Input: part model. Units: mm. Frame: model coordinates. A direction names the side the tool comes from. Coordinates: 2 decimals unless noted, no trailing zeros. Loops run counter-clockwise (first coordinate to the right, second up) from the corner with the lowest first, then second, coordinate; pieces in that order, holes last. Notation, with made-up numbers: (37.25, 82) - (77.25, 82) arc R29 cw to (77.25, 117) - close; hole circle Ø5 at (-34, 16.5). An arc over 180 degrees is marked (long way). Answer as CSV lines item,"result". Start each with the question number.
```python
from build123d import *

# Parameters (mm, degrees)
SKETCH1_W           = 40.2
SKETCH1_H           = 20.2
SKETCH1_W_2         = 38.2
SKETCH1_H_2         = 18.2
BOSS_EXTRUDE1_DEPTH = 10.65
FILLET1_R           = 1
SKETCH2_W           = 39.2
SKETCH2_H           = 19.2
SKETCH2_W_2         = 38.2
SKETCH2_H_2         = 18.2
BOSS_EXTRUDE2_DEPTH = 0.5
SKETCH3_W           = 38.2
SKETCH3_H           = 18.2
BOSS_EXTRUDE3_DEPTH = 1
BOSS_EXTRUDE4_START = -21.8
SKETCH4_R           = 1.4
BOSS_EXTRUDE4_DEPTH = 21.8
SKETCH5_R           = 1
CUT_EXTRUDE1_DEPTH  = 34.690677644
SKETCH6_W           = 40.2
SKETCH6_H           = 20.2
SKETCH6_W_2         = 39.2
SKETCH6_H_2         = 19.2
CUT_EXTRUDE2_DEPTH  = 2
SKETCH7_W           = 5
SKETCH7_H           = 2
CUT_EXTRUDE3_DEPTH  = 0.5


with BuildPart() as part:
    # Sketch1 → Boss-Extrude1 (new, symmetric)
    with BuildSketch(Plane(origin=(0, 0, 0), x_dir=(1, 0, 0), z_dir=(0, 1, 0))):
        with Locations((3.133727572, 0.855166052)):
            Rectangle(SKETCH1_W, SKETCH1_H)
        with Locations((3.133727572, 0.855166052)):
            Rectangle(SKETCH1_W_2, SKETCH1_H_2, mode=Mode.SUBTRACT)
    extrude(amount=BOSS_EXTRUDE1_DEPTH, both=True)

    # Fillet1
    fillet1_edges = [part.edges().sort_by_distance(p)[0] for p in [
        (-16.966272428, 0, -10.955166052),
        (23.233727572, 0, -10.955166052),
        (23.233727572, 0, 9.244833948),
        (-16.966272428, 0, 9.244833948),
    ]]
    fillet(fillet1_edges, radius=FILLET1_R)

    # Sketch2 → Boss-Extrude2 (add)
    with BuildSketch(Plane(origin=(0, 10.65, 0), x_dir=(1, 0, 0), z_dir=(0, 1, 0))):
        with Locations((3.133727572, 0.855166052)):
            Rectangle(SKETCH2_W, SKETCH2_H)
        with Locations((3.133727572, 0.855166052)):
            Rectangle(SKETCH2_W_2, SKETCH2_H_2, mode=Mode.SUBTRACT)
    extrude(amount=BOSS_EXTRUDE2_DEPTH)

    # Sketch3 → Boss-Extrude3 (add)
    with BuildSketch(Plane(origin=(0, 10.65, 0), x_dir=(1, 0, 0), z_dir=(0, 1, 0))):
        with Locations((3.133727572, 0.855166052)):
            Rectangle(SKETCH3_W, SKETCH3_H)
    extrude(amount=-BOSS_EXTRUDE3_DEPTH)

    # Sketch4 → Boss-Extrude4 (add)
    with BuildSketch(Plane(origin=(0, 11.15, 0), x_dir=(1, 0, 0), z_dir=(0, 1, 0)).offset(BOSS_EXTRUDE4_START)):
        with Locations((-15.066272428, 9.055166052)):
            Circle(SKETCH4_R)
        with Locations((-15.066272428, -7.344833948)):
            Circle(SKETCH4_R)
        with Locations((21.333727572, 9.055166052)):
            Circle(SKETCH4_R)
        with Locations((21.133727572, -7.344833948)):
            Circle(SKETCH4_R)
    extrude(amount=BOSS_EXTRUDE4_DEPTH)

    # Sketch5 → Cut-Extrude1 (cut, through all)
    with BuildSketch(Plane(origin=(0, 11.15, 0), x_dir=(1, 0, 0), z_dir=(0, 1, 0))):
        with Locations(Location((-15.066272428, 9.055166052, 0), (0, 0, 270))):
            Circle(SKETCH5_R)
        with Locations(Location((-15.066272428, -7.344833948, 0), (0, 0, 270))):
            Circle(SKETCH5_R)
        with Locations(Location((21.333727572, 9.055166052, 0), (0, 0, 270))):
            Circle(SKETCH5_R)
        with Locations(Location((21.133727572, -7.344833948, 0), (0, 0, 270))):
            Circle(SKETCH5_R)
    extrude(amount=-CUT_EXTRUDE1_DEPTH, mode=Mode.SUBTRACT)

    # Sketch6 → Cut-Extrude2 (cut)
    with BuildSketch(Plane.XZ.offset(10.65)):
        with Locations((3.133727572, -0.855166052)):
            Rectangle(SKETCH6_W, SKETCH6_H)
        with Locations((3.133727572, -0.855166052)):
            Rectangle(SKETCH6_W_2, SKETCH6_H_2, mode=Mode.SUBTRACT)
    extrude(amount=-CUT_EXTRUDE2_DEPTH, mode=Mode.SUBTRACT)

    # Sketch7 → Cut-Extrude3 (cut)
    with BuildSketch(Plane(origin=(22.733727572, 0, 0), x_dir=(0, 0, -1), z_dir=(1, 0, 0))):
        with Locations((0.755166052, -9.65)):
            Rectangle(SKETCH7_W, SKETCH7_H)
    extrude(amount=-CUT_EXTRUDE3_DEPTH, mode=Mode.SUBTRACT)


solid = part.part
```
Item 1: Draft query along X for faces 6 (the cylindrical face through (-14.1, 10.9, -8.04)), 7 (the flat face through (3.04, 11.15, -10.14)), 8 (the flat face through (3, -1, -9.955)), 9 (the cylindrical face through (-16.681, 0.865, -10.654)). Return one class per face: pulls with the +X half, pulls with the -X half, needs draft (parallel to the pull), parting line crosses it, or undercut.
Item 2: Section query C-C, the plane x = 16. Output: boundary loops of the cut face in (y, z), and give its area (3 significant figures).
Item 3: Section query B-B, the plane y = -9.5. Give the number of separate pieces and of enclosed holes in the cut face, and give its area (3 significant figures).
Item 4: Section query A-A, the plane z = -5.25. Output: boundary loops of the cut face in (x, y).
Item 5: Section query D-D, the plane z = -9.5. Output: boundary loops of the cut face in (x, y).
Item 6: Contact query for flat-ended pins moving along their axis: P1, Ø1.6, axis at y = -9.5, z = -8.5, coming from the +X side; P2, Ø2, axis at x = 10, z = 4, coming from the +Y side; P3, Ø0.6, axis at y = -10, z = 0, coming from the -X side; P4, Ø1.2, axis at x = 21.33, z = -9.06, coming from the -Y side. Output: stop coordinate, or through.
Item 7: Set-up query: faces 1 (the flat face through (3, -10, -10.455)), 2 (the flat face through (-16.966, 1, -1)), 3 (the flat face through (3, 1, -10.955)), 4 (the flat face through (-16.466, -10, -1)), 5 (the flat face through (22.234, -1, -1)). Return all of +Z, -Z, +X, -X, +Y, -Y with unobstructed straight access to the full face (end or side cutting, diameter ignored); none if empty.
Item 8: Material intervals for probe 1 along Z at (x, y) = (15.5, 5.75); probe 2 along X at (y, z) = (-6.75, -4); probe 3 along Z at (x, y) = (14.5, -9.5), sorted ascending.
Response values:
1,face 6,"undercut"
1,face 7,"needs draft"
1,face 8,"undercut"
1,face 9,"pulls with the -X half"
2,outline,"(-10.65, -10.46) - (-8.65, -10.46) - (-8.65, -10.96) - (10.65, -10.96) - (10.65, -10.46) - (11.15, -10.46) - (11.15, -9.96) - (10.65, -9.96) - (10.65, 8.24) - (11.15, 8.24) - (11.15, 8.74) - (10.65, 8.74) - (10.65, 9.24) - (-8.65, 9.24) - (-8.65, 8.74) - (-10.65, 8.74) - (-10.65, 8.24) - (9.65, 8.24) - (9.65, -9.96) - (-10.65, -9.96) - close"
2,area,"59.3 mm²"
3,separate pieces,"1"
3,enclosed holes,"5"
3,area,"61.4 mm²"
4,outline,"(-16.97, -8.65) - (-16.47, -8.65) - (-16.47, -10.65) - (-15.97, -10.65) - (-15.97, 9.65) - (22.23, 9.65) - (22.23, -10.65) - (22.73, -10.65) - (22.73, -8.65) - (23.23, -8.65) - (23.23, 10.65) - (22.73, 10.65) - (22.73, 11.15) - (22.23, 11.15) - (22.23, 10.65) - (-15.97, 10.65) - (-15.97, 11.15) - (-16.47, 11.15) - (-16.47, 10.65) - (-16.97, 10.65) - close"
5,outline,"(-16.97, -8.65) - (-16.47, -8.65) - (-16.47, -10.65) - (-15.96, -10.65) - (-15.96, 11.15) - (-16.47, 11.15) - (-16.47, 10.65) - (-16.97, 10.65) - close; (-14.17, -10.65) - (-13.74, -10.65) - (-13.74, 9.65) - (20.01, 9.65) - (20.01, -10.65) - (20.44, -10.65) - (20.44, 11.15) - (20.01, 11.15) - (20.01, 10.65) - (-13.74, 10.65) - (-13.74, 11.15) - (-14.17, 11.15) - close; (22.23, -10.65) - (22.73, -10.65) - (22.73, -8.65) - (23.23, -8.65) - (23.23, 10.65) - (22.73, 10.65) - (22.73, 11.15) - (22.23, 11.15) - close"
6,P1,"stops at x = 22.73"
6,P2,"stops at y = 10.65"
6,P3,"stops at x = -16.47"
6,P4,"passes through"
7,face 1,"-Z, +X, -X, -Y"
7,face 2,"+Z, -Z, -X, +Y, -Y"
7,face 3,"-Z, +X, -X, +Y, -Y"
7,face 4,"+Z, -Z, -X, -Y"
7,face 5,"-Y"
8,probe 1,"z = -10.96 to -9.96, 8.24 to 9.24"
8,probe 2,"x = -16.97 to -15.97, 22.23 to 23.23"
8,probe 3,"z = -10.46 to -9.96, 8.24 to 8.74"
